CAD build for the part. Positions are in the model's coordinates, mm. Face numbers are marked on the shaded views. A direction names the side the tool comes from. Give positions to 0.01 mm unless a question says otherwise; leave off trailing zeros. Write each loop counter-clockwise with the first axis right and the second up, starting at its lowest first coordinate (ties: lowest second). Pieces come first, ordered by that corner, then holes. Notation, with made-up numbers: (-2.5, 41.25) - (56.5, 41.25) arc R34 cw to (56.5, 74.25) - close; hole circle Ø9 at (63, 45). An arc over 180 degrees is marked (long way). Put each result on its own line as item: value. Start each with the question number.
1. Cut at A-A on z = 45. List the corners of the cut face in (x, y).
2. Tool access for the marked faces 1 and 2: list every direction of +Z, -Z, +X, -X, +Y, -Y with a clear straight run to the whole face (end or side of a thin tool).
3. Cut at C-C on y = 23. List the corners of the cut face in (x, z), and give its area (3 significant figures).
4. Mould opens along X. For the marked faces 3, 4 and 5 say: +X half, -X half, draft (parallel to the pull), parting line (faces both ways), or undercut.
5. Wall check: line 1 (X direction, y = 51.9, z = -45); line 2 (Y direction, x = 34.5, z = 46.5); line 3 (X direction, y = 23, z = -47). Give the ranges that are in metal, low to high.
6. Drop flat-ended pins along their axis: pin 1 (0.6 mm diameter, centred on y = 0, z = -4, fed in from -X); pin 2 (1.5 mm diameter, centred on x = -20.5, z = 17.5, fed in from -Y); pin 3 (18 mm diameter, centred on x = 10, y = 29, fed in from +Z); pin 4 (8 mm diameter, centred on x = -32, z = -26, fed in from +Y). Give the stop position or say it passes through.
7. Cut at D-D on x = 45. List the corners of the cut face in (y, z).
8. Cut at B-B on x = 10. List the corners of the cut face in (y, z).
from build123d import *

# Parameters (mm, degrees)
SKETCH1_R            = 1.6
BOSS_EXTRUDE1_DEPTH  = 1.5
BOSS_EXTRUDE10_DEPTH = 50
SKETCH5_R            = 10
CUT_EXTRUDE1_DEPTH   = 10
SKETCH6_R            = 1.6
BOSS_EXTRUDE11_DEPTH = 1
BOSS_EXTRUDE12_START = -1
BOSS_EXTRUDE12_DEPTH = 1


with BuildPart() as part:
    # Sketch1 → Boss-Extrude1 (new body)
    with BuildSketch(Plane(origin=(0, 0, 0), x_dir=(1, 0, 0), z_dir=(0, 1, 0))):
        with BuildLine():
            Line((48, -50), (-48, -50))
            ThreePointArc((-48, -50), (-49.414213562, -49.414213562), (-50, -48))
            Line((-50, -48), (-50, 48))
            ThreePointArc((-50, 48), (-49.414213562, 49.414213562), (-48, 50))
            Line((-48, 50), (48, 50))
            ThreePointArc((48, 50), (49.414213562, 49.414213562), (50, 48))
            Line((50, 48), (50, -48))
            ThreePointArc((50, -48), (49.414213562, -49.414213562), (48, -50))
        make_face()
        with Locations(Location((-45, 45, 0), (0, 0, 270))):
            Circle(SKETCH1_R, mode=Mode.SUBTRACT)
        with Locations(Location((45, 45, 0), (0, 0, 270))):
            Circle(SKETCH1_R, mode=Mode.SUBTRACT)
        with Locations(Location((45, -45, 0), (0, 0, 270))):
            Circle(SKETCH1_R, mode=Mode.SUBTRACT)
        with Locations(Location((-45, -45, 0), (0, 0, 270))):
            Circle(SKETCH1_R, mode=Mode.SUBTRACT)
    extrude(amount=BOSS_EXTRUDE1_DEPTH)



with BuildPart() as body_2:
    # Sketch2 → Boss-Extrude10 (new body)
    with BuildSketch(Plane(origin=(0, 1.5, 0), x_dir=(1, 0, 0), z_dir=(0, 1, 0))):
        with BuildLine():
            Line((48, 52), (-48, 52))
            ThreePointArc((-48, 52), (-50.828427125, 50.828427125), (-52, 48))
            Line((-52, 48), (-52, -48))
            ThreePointArc((-52, -48), (-50.828427125, -50.828427125), (-48, -52))
            Line((-48, -52), (48, -52))
            ThreePointArc((48, -52), (50.828427125, -50.828427125), (52, -48))
            Line((52, -48), (52, 48))
            ThreePointArc((52, 48), (50.828427125, 50.828427125), (48, 52))
        make_face()
        with BuildLine():
            Line((48, 50), (-48, 50))
            ThreePointArc((-48, 50), (-49.414213562, 49.414213562), (-50, 48))
            Line((-50, 48), (-50, -48))
            ThreePointArc((-50, -48), (-49.414213562, -49.414213562), (-48, -50))
            Line((-48, -50), (48, -50))
            ThreePointArc((48, -50), (49.414213562, -49.414213562), (50, -48))
            Line((50, -48), (50, 48))
            ThreePointArc((50, 48), (49.414213562, 49.414213562), (48, 50))
        make_face(mode=Mode.SUBTRACT)
    extrude(amount=BOSS_EXTRUDE10_DEPTH)

    # Sketch5 → Cut-Extrude1 (cut)
    with BuildSketch(Plane.XY.offset(52)):
        with Locations((10, 29)):
            Circle(SKETCH5_R)
    extrude(amount=-CUT_EXTRUDE1_DEPTH, mode=Mode.SUBTRACT)

    # Sketch6 → Boss-Extrude11 (add)
    with BuildSketch(Plane(origin=(0, 51.5, 0), x_dir=(1, 0, 0), z_dir=(0, 1, 0))):
        with BuildLine():
            Line((48, 52), (-48, 52))
            ThreePointArc((-48, 52), (-50.828427125, 50.828427125), (-52, 48))
            Line((-52, 48), (-52, -48))
            ThreePointArc((-52, -48), (-50.828427125, -50.828427125), (-48, -52))
            Line((-48, -52), (48, -52))
            ThreePointArc((48, -52), (50.828427125, -50.828427125), (52, -48))
            Line((52, -48), (52, 48))
            ThreePointArc((52, 48), (50.828427125, 50.828427125), (48, 52))
        make_face()
        with Locations(Location((-45, 45, 0), (0, 0, 270))):
            Circle(SKETCH6_R, mode=Mode.SUBTRACT)
        with Locations(Location((45, 45, 0), (0, 0, 270))):
            Circle(SKETCH6_R, mode=Mode.SUBTRACT)
        with Locations(Location((45, -45, 0), (0, 0, 270))):
            Circle(SKETCH6_R, mode=Mode.SUBTRACT)
        with Locations(Location((-45, -45, 0), (0, 0, 270))):
            Circle(SKETCH6_R, mode=Mode.SUBTRACT)
        with BuildLine():
            Line((-39, -41), (39, -41))
            ThreePointArc((39, -41), (40.414213562, -40.414213562), (41, -39))
            Line((41, -39), (41, 39))
            ThreePointArc((41, 39), (40.414213562, 40.414213562), (39, 41))
            Line((39, 41), (-39, 41))
            ThreePointArc((-39, 41), (-40.414213562, 40.414213562), (-41, 39))
            Line((-41, 39), (-41, -39))
            ThreePointArc((-41, -39), (-40.414213562, -40.414213562), (-39, -41))
        make_face(mode=Mode.SUBTRACT)
    extrude(amount=BOSS_EXTRUDE11_DEPTH)


with BuildPart() as part_1:
    add(part.part)

    add(body_2.part)  # Boss-Extrude12 merges body 2
    # Sketch2_6 → Boss-Extrude12 (add)
    with BuildSketch(Plane(origin=(0, 1.5, 0), x_dir=(1, 0, 0), z_dir=(0, 1, 0)).offset(BOSS_EXTRUDE12_START)):
        with BuildLine():
            Line((48, 52), (-48, 52))
            ThreePointArc((-48, 52), (-50.828427125, 50.828427125), (-52, 48))
            Line((-52, 48), (-52, -48))
            ThreePointArc((-52, -48), (-50.828427125, -50.828427125), (-48, -52))
            Line((-48, -52), (48, -52))
            ThreePointArc((48, -52), (50.828427125, -50.828427125), (52, -48))
            Line((52, -48), (52, 48))
            ThreePointArc((52, 48), (50.828427125, 50.828427125), (48, 52))
        make_face()
        with BuildLine():
            Line((48, 50), (-48, 50))
            ThreePointArc((-48, 50), (-49.414213562, 49.414213562), (-50, 48))
            Line((-50, 48), (-50, -48))
            ThreePointArc((-50, -48), (-49.414213562, -49.414213562), (-48, -50))
            Line((-48, -50), (48, -50))
            ThreePointArc((48, -50), (49.414213562, -49.414213562), (50, -48))
            Line((50, -48), (50, 48))
            ThreePointArc((50, 48), (49.414213562, 49.414213562), (48, 50))
        make_face(mode=Mode.SUBTRACT)
    extrude(amount=BOSS_EXTRUDE12_DEPTH)


solid = part_1.part
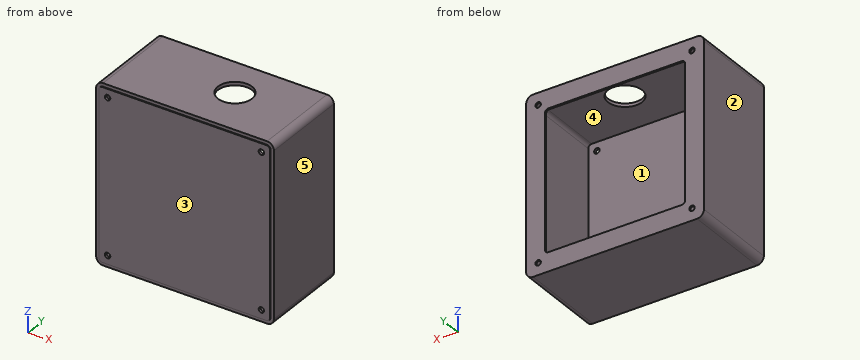
Report:
1. outline: (-52, 0.5) - (-50, 0.5) - (-50, 0) - (-46.6, 0) - (-46.6, 1.5) - (-50, 1.5) - (-50, 51.5) - (-46.6, 51.5) - (-46.6, 52.5) - (-52, 52.5) - close; (-43.4, 0) - (43.4, 0) - (43.4, 1.5) - (-43.4, 1.5) - close; (-43.4, 51.5) - (43.4, 51.5) - (43.4, 52.5) - (-43.4, 52.5) - close; (46.6, 0) - (50, 0) - (50, 0.5) - (52, 0.5) - (52, 52.5) - (46.6, 52.5) - (46.6, 51.5) - (50, 51.5) - (50, 1.5) - (46.6, 1.5) - close
2. face 1: none
2. face 2: +Z, -Z, -X, +Y, -Y
3. outline: (-52, -48) arc R4 ccw to (-48, -52) - (48, -52) arc R4 ccw to (52, -48) - (52, 48) arc R4 ccw to (48, 52) - (18, 52) - (18, 50) - (48, 50) arc R2 cw to (50, 48) - (50, -48) arc R2 cw to (48, -50) - (-48, -50) arc R2 cw to (-50, -48) - (-50, 48) arc R2 cw to (-48, 50) - (2, 50) - (2, 52) - (-48, 52) arc R4 ccw to (-52, 48) - close
3. area: 774 mm²
4. face 3: draft
4. face 4: undercut
4. face 5: +X half
5. line 1: x = -52 to -46.6, -43.4 to 43.4, 46.6 to 52
5. line 2: y = 0 to 1.5, 51.5 to 52.5
5. line 3: x = -52 to -50, 50 to 52
6. pin 1: stops at x = -50
6. pin 2: stops at y = 0
6. pin 3: stops at z = -50
6. pin 4: stops at y = 1.5
7. outline: (0, -50) - (0.5, -50) - (0.5, -52) - (52.5, -52) - (52.5, -46.6) - (51.5, -46.6) - (51.5, -50) - (1.5, -50) - (1.5, -46.6) - (0, -46.6) - close; (0, -43.4) - (1.5, -43.4) - (1.5, 43.4) - (0, 43.4) - close; (0, 46.6) - (1.5, 46.6) - (1.5, 50) - (51.5, 50) - (51.5, 46.6) - (52.5, 46.6) - (52.5, 52) - (0.5, 52) - (0.5, 50) - (0, 50) - close; (51.5, -43.4) - (52.5, -43.4) - (52.5, 43.4) - (51.5, 43.4) - close
8. outline: (0, -50) - (0.5, -50) - (0.5, -52) - (52.5, -52) - (52.5, -41) - (51.5, -41) - (51.5, -50) - (1.5, -50) - (1.5, 50) - (19, 50) - (19, 52) - (0.5, 52) - (0.5, 50) - (0, 50) - close; (39, 50) - (51.5, 50) - (51.5, 41) - (52.5, 41) - (52.5, 52) - (39, 52) - close
